Geometry check sheet. Reference: the model listing, model coordinates, mm. Give positions to 0.01 mm unless a question says otherwise; leave off trailing zeros. Loops run counter-clockwise (first coordinate to the right, second up) from the corner with the lowest first, then second, coordinate; pieces in that order, holes last. Notation, with made-up numbers: (83, -12) -> (121, -12) arc R34 ccw to (121, 24) -> close; hole circle Ø2 at (41.5, -15.75). An arc over 180 degrees is marked (long way). Write each question's results on one line, items separated by ' | '. Start each with the question number.
1) Scan lines: line 1 (Y direction, x = 147, z = 1.5); line 2 (Z direction, x = 52, y = 4); line 3 (Z direction, x = 157, y = 3.5). Record each from-to range of solid material in increasing order. Write a range as from..to.
2) Sectioned sample at B-B on x = 141.5. Record the cut outline in (y, z), then the cut area to 3 significant figures.
3) Depth check by flat-ended pin: pin 1 (1.9 mm diameter, centred on x = 88.5, z = 8, fed in from -Y); pin 2 (4.5 mm diameter, centred on x = 148, y = 3.5, fed in from +Z); pin 3 (4 mm diameter, centred on x = 57, y = 4, fed in from +Z); pin 4 (4 mm diameter, centred on x = 147, y = 4, fed in from +Z). Enter the tip coordinate at first touch or a pass-through.
4) Sectioned sample at A-A on x = 99. Record the cut outline in (y, z).
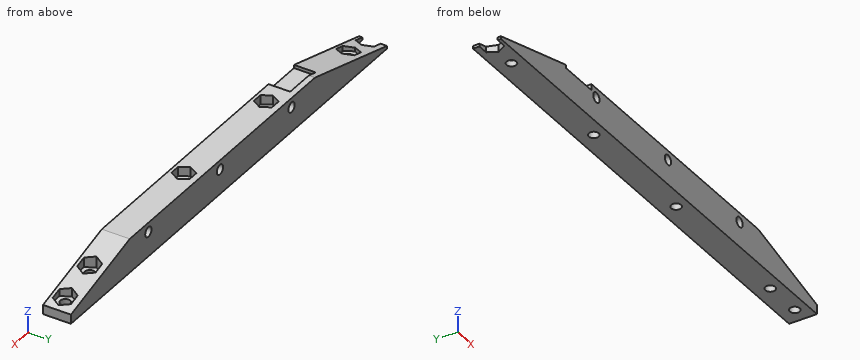
Autodesk Inventor part; units mm, degrees
ref_plane "YZ Plane" through (0, 0, 0) normal (1, 0, 0) x (0, 1, 0)
ref_plane "XZ Plane" through (0, 0, 0) normal (0, 1, 0) x (-1, 0, 0)
ref_plane "XY Plane" through (0, 0, 0) normal (0, 0, 1) x (1, 0, 0)
sketch "Sketch1" plane through (0, 0, 0) normal (0, 0, 1) x (1, 0, 0)
  line L0 (0, 0) -> (164.5, 0)
  line L1 (164.5, 0) -> (164.5, 9)
  line L2 (164.5, 9) -> (0, 9)
  line L3 (0, 9) -> (0, 0)
  circle A0 centre (57, 4) radius 1.6
  circle A1 centre (99, 4) radius 1.6
  circle A2 centre (159.5, 4) radius 1.6
  circle A3 centre (147, 4) radius 1.6
  circle A4 centre (15, 4) radius 1.6
  circle A5 centre (5, 4) radius 1.6
  dimension "d1" = 9
  dimension "d2" = 90
  dimension "d4" = 3.2
  dimension "d6" = 3.2
  dimension "d7" = 3.2
  dimension "d8" = 42
  dimension "d9" = 60.5
  dimension "d26" = 3.2
  dimension "d27" = 48
  dimension "d28" = 3.2
  dimension "d29" = 42
  dimension "d32" = 15
  dimension "d33" = 5
  dimension "d61" = 3.2
  dimension "d62" = 10
  dimension "d63" = 12.5
  dimension "d108" = 4
  dimension "d109" = 4
  dimension "d110" = 4
  dimension "d111" = 4
  dimension "d112" = 4
  dimension "d113" = 4
ref_plane "Work Plane2" through (0, 0, 0) normal (0, -1, 0) x (1, 0, 0)
sketch "Sketch2" plane through (0, 0, 0) normal (0, -1, 0) x (1, 0, 0)
  circle A0 centre (52, 8) radius 1.6
  circle A1 centre (125, 8) radius 1.6
  circle A2 centre (88.5, 8) radius 1.6
  point P0 (0, 0)
  point P1 (52, 0)
  dimension "d13" = 3.2
  dimension "d15" = 3.2
  dimension "d17" = 3.2
  dimension "d18" = 36.5
  dimension "d64" = 52
  dimension "d65" = 36.5
  dimension "d114" = 8
  dimension "d115" = 73
ref_plane "Work Plane1" through (0, 0, 11) normal (0, 0, 1) x (1, 0, 0)
extrude "klocek" add sketch "Sketch1" along normal blind 11
ref_plane "Work Plane3" through (0, 0, 0) normal (0, -1, 0) x (1, 0, 0)
extrude "prowadzenie osi" cut sketch "Sketch2" against normal up to next
ref_plane "Work Plane4" through (0, 0, 0) normal (0, -1, 0) x (1, 0, 0)
sketch "Sketch7" plane through (0, 0, 0) normal (0, -1, 0) x (1, 0, 0)
  line L0 (0, 11) -> (0, 0)
  line L1 (0, 11) -> (164.5, 11)
  line L2 (0, 11) -> (40, 11)
  line L3 (40, 11) -> (0, 0)
  point P0 (0, -1.8333)
  dimension "d86" = 11
  dimension "d87" = 40
sketch "Sketch8" plane through (0, 0, 0) normal (0, -1, 0) x (1, 0, 0)
  line L0 (164.5, 0) -> (164.5, 11)
  line L1 (164.5, 11) -> (164.5, 3)
  line L2 (164.5, 11) -> (0, 11)
  line L3 (164.5, 11) -> (134.5, 11)
  line L4 (134.5, 11) -> (164.5, 3)
  point P0 (0, 0)
  point P1 (40.8333, 11)
  dimension "d80" = 8
  dimension "d81" = 30
extrude "przedni skos" cut sketch "Sketch7" against normal up to next
extrude "tylni skos" cut sketch "Sketch8" against normal up to next
ref_plane "Work Plane7" through (0, 0, 11) normal (0, 0, 1) x (1, 0, 0)
sketch "Sketch5" plane through (0, 0, 11) normal (0, 0, 1) x (1, 0, 0)
  circle A0 centre (99, 4) radius 1.6
  line L0 (95.5936, 4) -> (97.2968, 6.95)
  line L1 (97.2968, 6.95) -> (100.7032, 6.95)
  line L2 (100.7032, 6.95) -> (102.4064, 4)
  line L3 (102.4064, 4) -> (100.7032, 1.05)
  line L4 (100.7032, 1.05) -> (97.2968, 1.05)
  line L5 (97.2968, 1.05) -> (95.5936, 4)
  circle A1 centre (57, 4) radius 1.6
  line L6 (60.4064, 4) -> (58.7032, 1.05)
  line L7 (58.7032, 1.05) -> (55.2968, 1.05)
  line L8 (55.2968, 1.05) -> (53.5936, 4)
  line L9 (53.5936, 4) -> (55.2968, 6.95)
  line L10 (55.2968, 6.95) -> (58.7032, 6.95)
  line L11 (58.7032, 6.95) -> (60.4064, 4)
  point P0 (119.5, 5)
  dimension "d98" = 5.9
  dimension "d100" = 5.9
extrude "hex insert middle" cut sketch "Sketch5" against normal blind 3
ref_plane "Work Plane6" through (0, 0, 11) normal (0, 0, 1) x (1, 0, 0)
sketch "Sketch9" plane through (0, 0, 11) normal (0, 0, 1) x (1, 0, 0)
  circle A0 centre (147, 4) radius 1.6
  line L0 (150.4064, 4) -> (148.7032, 1.05)
  line L1 (148.7032, 1.05) -> (145.2968, 1.05)
  line L2 (145.2968, 1.05) -> (143.5936, 4)
  line L3 (143.5936, 4) -> (145.2968, 6.95)
  line L4 (145.2968, 6.95) -> (148.7032, 6.95)
  line L5 (148.7032, 6.95) -> (150.4064, 4)
  point P0 (0, 0)
  point P1 (153, 5)
  dimension "d99" = 5.9
extrude "hex insert rear 1" cut sketch "Sketch9" against normal blind 6
ref_plane "Work Plane5" through (0, 0, 11) normal (0, 0, 1) x (1, 0, 0)
sketch "Sketch10" plane through (0, 0, 11) normal (0, 0, 1) x (1, 0, 0)
  circle A0 centre (159.5, 4) radius 1.6
  line L0 (162.9064, 4) -> (161.2032, 1.05)
  line L1 (161.2032, 1.05) -> (157.7968, 1.05)
  line L2 (157.7968, 1.05) -> (156.0936, 4)
  line L3 (156.0936, 4) -> (157.7968, 6.95)
  line L4 (157.7968, 6.95) -> (161.2032, 6.95)
  line L5 (161.2032, 6.95) -> (162.9064, 4)
  point P0 (0, 0)
  dimension "d101" = 5.9
extrude "hex insert rear 2" cut sketch "Sketch10" against normal blind 8.5
sketch "Sketch13" plane through (0, 0, 11) normal (0, 0, 1) x (1, 0, 0)
  circle A0 centre (5, 4) radius 1.6
  line L0 (8.4064, 4) -> (6.7032, 1.05)
  line L1 (6.7032, 1.05) -> (3.2968, 1.05)
  line L2 (3.2968, 1.05) -> (1.5936, 4)
  line L3 (1.5936, 4) -> (3.2968, 6.95)
  line L4 (3.2968, 6.95) -> (6.7032, 6.95)
  line L5 (6.7032, 6.95) -> (8.4064, 4)
  point P0 (0, 0)
  dimension "d90" = 5.9
extrude "hex insert front 1" cut sketch "Sketch13" against normal through all
sketch "Sketch16" plane through (0, 0, 11) normal (0, 0, 1) x (1, 0, 0)
  circle A0 centre (15, 4) radius 1.6
  line L0 (18.4064, 4) -> (16.7032, 1.05)
  line L1 (16.7032, 1.05) -> (13.2968, 1.05)
  line L2 (13.2968, 1.05) -> (11.5936, 4)
  line L3 (11.5936, 4) -> (13.2968, 6.95)
  line L4 (13.2968, 6.95) -> (16.7032, 6.95)
  line L5 (16.7032, 6.95) -> (18.4064, 4)
  point P0 (0, 0)
  dimension "d93" = 5.9
extrude "hex insert front 2" cut sketch "Sketch16" against normal blind 9
sketch "Sketch17" plane through (0, 0, 0) normal (0, 0, -1) x (-1, 0, 0)
  line L0 (0, 9) -> (0, 0)
  line L1 (0, 0) -> (-3.2968, 0)
  line L2 (-3.2968, 0) -> (-3.2968, 10.0042)
  line L3 (-3.2968, 10.0042) -> (0, 10.0042)
  line L4 (0, 10.0042) -> (0, 0)
extrude "Extrusion20" cut sketch "Sketch17" against normal up to next
sketch "Sketch18" plane through (40, 0, 11) normal (0, -1, 0) x (1, 0, 0)
  line L0 (9.5, 0) -> (9.5, -2)
  line L1 (9.5, -2) -> (-3.5, -2)
  line L2 (-3.5, -2) -> (-3.5, 0)
  line L3 (-3.5, 0) -> (9.5, 0)
  line L4 (94.5, 0) -> (0, 0)
  circle A0 centre (12, -3) radius 1.6
  line L5 (-36.7032, -11) -> (124.5, -11)
  point P0 (-40, -11)
  dimension "d102" = 2
  dimension "d103" = 13
  dimension "d104" = 2.5
extrude "Extrusion21" cut sketch "Sketch18" against normal blind 7 contours L0 L1 L2 L3
properties part number "wheel_support_v2_narrow_with_line_sensor"
Result:
1) line 1: 0..2.4, 5.6..9 | line 2: 0..6.4, 9.6..11 | line 3: 0..2.5
2) outline: (0, 0) -> (9, 0) -> (9, 9.13) -> (0, 9.13) -> close | area: 82.2 mm^2
3) pin 1: through | pin 2: z = 7.15 | pin 3: z = 8 | pin 4: z = 5
4) outline: (0, 0) -> (2.4, 0) -> (2.4, 8) -> (1.05, 8) -> (1.05, 11) -> (0, 11) -> close; (5.6, 0) -> (9, 0) -> (9, 11) -> (6.95, 11) -> (6.95, 8) -> (5.6, 8) -> close
